```python
from build123d import *

# Parameters (mm, degrees)
F0_R     = 290
F1_DEPTH = 880
F2_W     = 250
F2_H     = 680
F3_DEPTH = 566
F4_T     = -1
F5_R     = 50
F6_DEPTH = 314


with BuildPart() as f1:
    # F0 (on Front) → F1 (new body)
    with BuildSketch(Plane.XZ):
        Circle(F0_R)
    extrude(amount=F1_DEPTH)

    # F2 (on Top) → F3 (cut)
    with BuildSketch(Plane.XY):
        with Locations((-125, -440)):
            Rectangle(F2_W, F2_H)
    extrude(amount=F3_DEPTH, mode=Mode.SUBTRACT)

    # F4
    f4_openings = [f1.faces().sort_by_distance(p)[0] for p in [
        (0, -440, 145),
        (-250, -440, 73.484692),
        (-125, -440, 0),
        (-113.917816, -780, 127.398954),
        (-113.917816, -100, 127.398954),
    ]]
    offset(amount=F4_T, openings=f4_openings)

    # F5 (on Top) → F6 (cut)
    with BuildSketch(Plane.XY):
        with Locations((216.3317799568, -116.8923303485)):
            Circle(F5_R)
    extrude(amount=F6_DEPTH, mode=Mode.SUBTRACT)


solid = f1.part
```
Work out the finished part from the listing and answer in its coordinate system (mm). A direction names the side the tool comes from. Give positions to 0.01 mm unless a question says otherwise; leave off trailing zeros. Write each loop counter-clockwise with the first axis right and the second up, starting at its lowest first coordinate (ties: lowest second). Pieces come first, ordered by that corner, then holes. Notation, with made-up numbers: (62.5, 16) -> (114.5, 16) arc R23 ccw to (114.5, 42) -> close; hole circle Ø2 at (63.5, 43.5). An arc over 180 degrees is marked (long way). Write each question's results on one line, items separated by ' | '.
1. Straight lines are drawn through the part: L1, parallel to Y at x = 52, z = -240.5; L2, parallel to X at y = -290, z = -9; L3, parallel to X at y = -276.5, z = 34. For each, find the intervals that lie inside material, in ascending order.
Data:
L1: -880 to -879, -1 to 0 | L2: -289.86 to -288.86, 288.86 to 289.86 | L3: -288 to -286.99, 286.99 to 288
2. Find section D-D on y = -626. Determine the outline of the cut face in (x, z), and give its area (3 significant figures).
Data:
outline: (-250, 144.99) -> (-250, 146.97) arc R290 ccw (long way) to (0, 290) -> (0, 289) arc R289 cw (long way) to start | area: 1,520 mm^2
3. Find section C-C on x = 186. Determine the outline of the cut face in (y, z).
Data:
outline: (-880, -222.49) -> (0, -222.49) -> (0, 222.49) -> (-77.14, 222.49) -> (-77.14, 221.19) -> (-1, 221.19) -> (-1, -221.19) -> (-879, -221.19) -> (-879, 221.19) -> (-156.64, 221.19) -> (-156.64, 222.49) -> (-880, 222.49) -> close
4. Find section B-B on x = 82.5. Determine the outline of the cut face in (y, z), and give its area (3 significant figures).
Data:
outline: (-880, -278.02) -> (0, -278.02) -> (0, 278.02) -> (-880, 278.02) -> close; hole (-879, -276.97) -> (-1, -276.97) -> (-1, 276.97) -> (-879, 276.97) -> close | area: 2,940 mm^2
5. Each of these flat-tipped pins is pushed along its axis until it touches: pin 1 Ø8 at (y, z) = (-444, 61.5) entering from -X; pin 2 Ø0.5 at (y, z) = (-585, 289.5) entering from -X; pin 3 Ø10 at (y, z) = (-149, -205.5) entering from +X. Where does it stop, or does it pass through?
Data:
pin 1: x = -284.24 | pin 2: x = 0 | pin 3: x = 209.52
6. Find section A-A on z = 0. Determine the outline of the cut face in (x, y).
Data:
outline: (-290, -880) -> (290, -880) -> (290, 0) -> (-290, 0) -> close; hole (-289, -879) -> (289, -879) -> (289, -1) -> (-289, -1) -> close
7. A tool of negligible diameter and unlimited length cuts with its end or side. For faces 4 (the flat face through (-4, -879, 4)), 5 (the flat face through (-4, 0, 4)), from which of +Z, -Z, +X, -X, +Y, -Y can it reach the whole face along a straight path? Write none if from no direction.
Data:
face 4: none | face 5: +Z, -Z, +X, -X, +Y
8. Determine the mould class of faces 1 (the cylindrical face through (133.82, -433.84, -257.28)), 2 (the cylindrical face through (133.36, -433.85, -256.39)), 3 (the flat face through (-4, -880, 4)) for opening direction Z: +Z half, -Z half, draft (parallel to the pull), parting line (faces both ways), or undercut.
Data:
face 1: parting line | face 2: undercut | face 3: draft
